from build123d import *

# Parameters (mm, degrees)
POCKET010_DEPTH  = 10.5
HOLE_D           = 3.9
HOLE_DEPTH       = 25
HOLE_CBORE_D     = 6.7
HOLE_CBORE_DEPTH = 14
HOLE_TIPS_R      = 1.95


with BuildPart() as part:
    # Sketch022 → AdditiveLoft001 section 0
    with BuildSketch(Plane.XZ.offset(26)):
        with BuildLine():
            Line((-24.5, 0), (33.5, 0))
            Line((33.5, 0), (39.5, -6.5))
            Line((39.5, -6.5), (42.439214, -3.78688))
            ThreePointArc((42.439214, -3.78688), (-2.100464, 12.941774), (-44.952563, -7.730146))
            Line((-44.952563, -7.730146), (-41.5, -9.75))
            ThreePointArc((-24.5, 0), (-34.298756, -2.610502), (-41.5, -9.75))
        make_face()
    # Sketch023 → AdditiveLoft001 section 1
    with BuildSketch(Plane.XZ):
        with BuildLine():
            Line((-24.5, 0), (33.5, 0))
            Line((33.5, 0), (39.5, -6.5))
            Line((39.5, -6.5), (42.439214, -3.78688))
            ThreePointArc((42.439214, -3.78688), (-1.784428, 5.937707), (-44.952563, -7.730146))
            Line((-44.952563, -7.730146), (-41.5, -9.75))
            ThreePointArc((-24.5, 0), (-34.298756, -2.610502), (-41.5, -9.75))
        make_face()
    loft()

    # Sketch024 → Pocket010 (cut, symmetric)
    with BuildSketch(Plane.XY):
        with BuildLine():
            Line((-22, 0), (9.990911, -0.825847))
            Line((9.990911, -0.825847), (33.005764, -3.416537))
            Line((33.005764, -3.416537), (43.190086, -13.274679))
            Line((43.190086, -13.274679), (43.190086, 17.224566))
            Line((43.190086, 17.224566), (-48.844296, 17.224566))
            Line((-48.844296, 17.224566), (-48.844296, -33.398815))
            Line((-48.844296, -33.398815), (-45, -33.398815))
            Line((-45, -33.398815), (-45, -26))
            add(Edge.make_bspline(
                [(-45, -26), (-42.180007, 0.520948), (-22, 0)],
                knots=[-21.613822, -21.613822, -21.613822, 11.787032, 11.787032, 11.787032], degree=2))
        make_face()
    extrude(amount=POCKET010_DEPTH, both=True, mode=Mode.SUBTRACT)

    # Hole
    with Locations(Plane.XY.offset(17)):
        with Locations((0, -21)):
            CounterBoreHole(HOLE_D / 2, HOLE_CBORE_D / 2, HOLE_CBORE_DEPTH, depth=HOLE_DEPTH)

    # Hole tips → Hole tip 1 section 0
    with BuildSketch(Plane.XY.offset(-8), mode=Mode.PRIVATE) as hole_tip_1_s0:
        with Locations((0, -21)):
            Circle(HOLE_TIPS_R)
    loft([hole_tip_1_s0.sketch, Vertex(0, -21, -9.171678)], mode=Mode.SUBTRACT)


solid = part.part
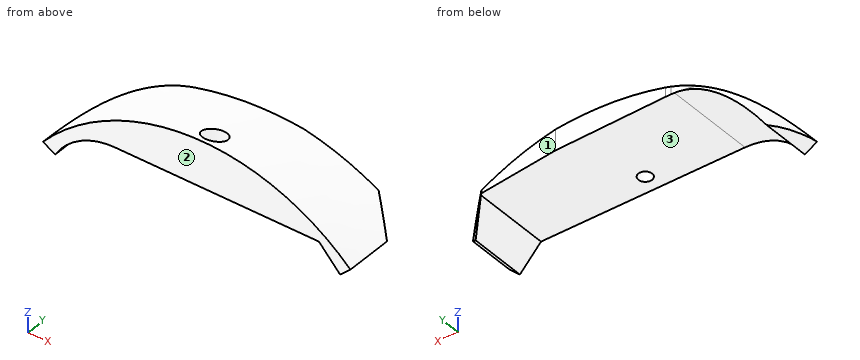
Part model, mm, in its own coordinate system. Face numbers are marked on the shaded views. Give positions to 0.01 mm unless a question says otherwise; leave off trailing zeros. One line per question, with ' | ' between items.
1. Drop flat-ended pins along their axis: P1, Ø1.5, axis at x = 13.5, z = -1, coming from the +Y side; P2, Ø6, axis at x = 25, y = -21.5, coming from the +Z side; P3, Ø5, axis at x = 0, y = -21, coming from the -Z side; P4, Ø2, axis at y = -12, z = 4.5, coming from the -X side. Give the stop position or say it passes through.
Filled in:
P1: through | P2: z = 8.32 | P3: z = 0 | P4: x = -26.84
2. Drill centre lines: probe 1 along Y at (x, z) = (0, 5.5); probe 2 along Y at (x, z) = (0, 1.35); probe 3 along X at (y, z) = (-2.5, -1.5). Where is each one in solid material? Low to high.
Filled in:
probe 1: -26 to -24.35, -17.65 to -0.57 | probe 2: -26 to -22.95, -19.05 to -0.57 | probe 3: -33.25 to -32.04
3. Pull direction X, two halves, no side cores. Call the marked faces 1, 2 and 3: +X half, -X half, draft (parallel to the pull), parting line (faces both ways), or undercut.
Filled in:
face 1: +X half | face 2: draft | face 3: undercut
